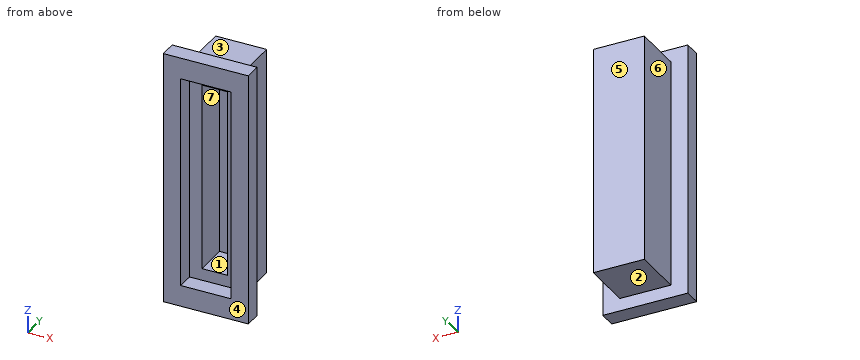
from build123d import *

# Parameters (mm, degrees)
SKETCH_1_W          = 6
SKETCH_1_H          = 27
SKETCH_1_W_2        = 3
SKETCH_1_H_2        = 22.2
EXTRUDE_1_DEPTH     = 4
SKETCH_2_W          = 6
SKETCH_2_H          = 27
EXTRUDE_2_DEPTH     = 2
SKETCH_3_W          = 10
SKETCH_3_H          = 30
EXTRUDE_3_DEPTH     = 2
SKETCH_4_W          = 5.9
SKETCH_4_H          = 25
CUT_EXTRUDE_3_DEPTH = 2


with BuildPart() as part:
    # 草图1 → 凸台-拉伸1 (new body)
    with BuildSketch(Plane(origin=(0, 0, 0), x_dir=(1, 0, 0), z_dir=(0, 1, 0))):
        Rectangle(SKETCH_1_W, SKETCH_1_H)
        Rectangle(SKETCH_1_W_2, SKETCH_1_H_2, mode=Mode.SUBTRACT)
    extrude(amount=EXTRUDE_1_DEPTH)

    # 草图2 → 凸台-拉伸2 (add)
    with BuildSketch(Plane(origin=(0, 4, 0), x_dir=(1, 0, 0), z_dir=(0, 1, 0))):
        Rectangle(SKETCH_2_W, SKETCH_2_H)
    extrude(amount=EXTRUDE_2_DEPTH)

    # 草图3 → 凸台-拉伸3 (add)
    with BuildSketch(Plane.XZ):
        Rectangle(SKETCH_3_W, SKETCH_3_H)
    extrude(amount=EXTRUDE_3_DEPTH)

    # 草图4 → 切除-拉伸3 (cut)
    with BuildSketch(Plane.XZ.offset(2)):
        Rectangle(SKETCH_4_W, SKETCH_4_H)
    extrude(amount=-CUT_EXTRUDE_3_DEPTH, mode=Mode.SUBTRACT)


solid = part.part
Model file for the job. Use its own axes, mm. Face numbers are marked on the shaded views. A direction names the side the tool comes from. Give positions to 0.01 mm unless a question says otherwise; leave off trailing zeros. Order: outer loops, then holes, each group sorted by start corner. A loop starts at its lowest first (then second) coordinate and runs counter-clockwise, first axis right, second up. Notation, with made-up numbers: (86, -24) -> (124, -24) arc R22 ccw to (124, 13) -> close; hole circle Ø10 at (51, -5). An arc over 180 degrees is marked (long way). Use CSV: the item, a comma, the result in double quotes.
1. Band-saw the part on D-D, the plane y = 5. Give the cut face in (x, z).
Outcome:
outline,"(-3, -13.5) -> (3, -13.5) -> (3, 13.5) -> (-3, 13.5) -> close"
2. Mould opens along X. For the marked faces 5, 6 and 7 say: +X half, -X half, draft (parallel to the pull), parting line (faces both ways), or undercut.
Outcome:
face 5,"draft"
face 6,"-X half"
face 7,"undercut"
3. Drop flat-ended pins along their axis: pin 1 (0.9 mm diameter, centred on x = 0, z = 4, fed in from -Y); pin 2 (1.5 mm diameter, centred on x = -2, y = 2.5, fed in from -Z); pin 3 (0.9 mm diameter, centred on x = -0.5, y = 1, fed in from +Z). Give the stop position or say it passes through.
Outcome:
pin 1,"y = 4"
pin 2,"z = -13.5"
pin 3,"z = 13.5"
4. Drill centre lines: line 1 along X through (y, z) = (-1.5, 3.5); line 2 along X through (y, z) = (3.75, -4.5); line 3 along Z through (x, y) = (-0.5, 3). Where is each one in solid material? Low to high. Write a range as from..to.
Outcome:
line 1,"-5..-2.95, 2.95..5"
line 2,"-3..-1.5, 1.5..3"
line 3,"-13.5..-11.1, 11.1..13.5"
5. Band-saw the part on B-B, the plane x = 1. Give the cut face in (y, z), then the cut area to 3 significant figures.
Outcome:
outline,"(-2, -15) -> (0, -15) -> (0, -13.5) -> (6, -13.5) -> (6, 13.5) -> (0, 13.5) -> (0, 15) -> (-2, 15) -> (-2, 12.5) -> (0, 12.5) -> (0, 11.1) -> (4, 11.1) -> (4, -11.1) -> (0, -11.1) -> (0, -12.5) -> (-2, -12.5) -> close"
area,"83.2 mm²"
6. Band-saw the part on C-C, the plane z = -0.5. Give the cut face in (x, y).
Outcome:
outline,"(-5, -2) -> (-2.95, -2) -> (-2.95, 0) -> (-1.5, 0) -> (-1.5, 4) -> (1.5, 4) -> (1.5, 0) -> (2.95, 0) -> (2.95, -2) -> (5, -2) -> (5, 0) -> (3, 0) -> (3, 6) -> (-3, 6) -> (-3, 0) -> (-5, 0) -> close"
7. 3-axis set-ups, long thin cutter, end or side, ignore diameter. For the marked faces 1, 2, 3 and 4: which of +Z, -Z, +X, -X, +Y, -Y reach the whole face in a straight line?
Outcome:
face 1,"-Y"
face 2,"-Z, +X, -X, +Y"
face 3,"+Z, +X, -X, +Y"
face 4,"+Z, -Z, +X, -X, -Y"
8. Band-saw the part on A-A, the plane y = 1.75. Give the cut face in (x, z), then the cut area to 3 significant figures.
Outcome:
outline,"(-3, -13.5) -> (3, -13.5) -> (3, 13.5) -> (-3, 13.5) -> close; hole (-1.5, -11.1) -> (1.5, -11.1) -> (1.5, 11.1) -> (-1.5, 11.1) -> close"
area,"95.4 mm²"
